Drawing for the job (mm, zero at the part's lowest x, y, z). A direction names the side the tool comes from. Coordinates: 2 decimals unless noted, no trailing zeros. Write each loop counter-clockwise with the first axis right and the second up, starting at its lowest first coordinate (ties: lowest second). Pieces come first, ordered by that corner, then holes. Notation, with made-up numbers: M 56,-28 L 72,-28 A9 ccw 72,-22 Z; hole C 71,1 d4. An arc over 180 degrees is marked long. Put each result on its own line as item: value. Start each with the question number.
Q1. Cut at C-C (y = 3.5). Write the cut outline in (x, z), then the cut area to 3 significant figures.
Q2. Drill centre lines: line 1 along X through (y, z) = (2, 1.75); line 2 along Y through (x, z) = (11.75, 6.5); line 3 along X through (y, z) = (5.75, 5). Where is each one in solid material? Low to high.
Q3. Drop flat-ended pins along their axis: pin 1 (0.6 mm diameter, centred on x = 1, y = 0.5, fed in from -Z); pin 2 (0.6 mm diameter, centred on x = 13.5, z = 9, fed in from +Y); pin 3 (0.8 mm diameter, centred on x = 10, y = 6, fed in from +Z); pin 4 (1.5 mm diameter, centred on y = 1, z = 8.5, fed in from -X). Give the stop position or say it passes through.
Q4. Cut at D-D (z = 8.75). Write the cut outline in (x, y).
Q5. Cut at A-A (x = 13). Write the cut outline in (y, z), then the cut area to 3 significant figures.
Q6. Cut at B-B (z = 2.25). Write the cut outline in (x, y), then the cut area to 3 significant figures.
Q7. Which spindle directions (+Z, -Z, +X, -X, +Y, -Y) get a long thin tool onto all of the face, cutting with end or side? Do the marked faces 1 and 2. Say none if no direction does.
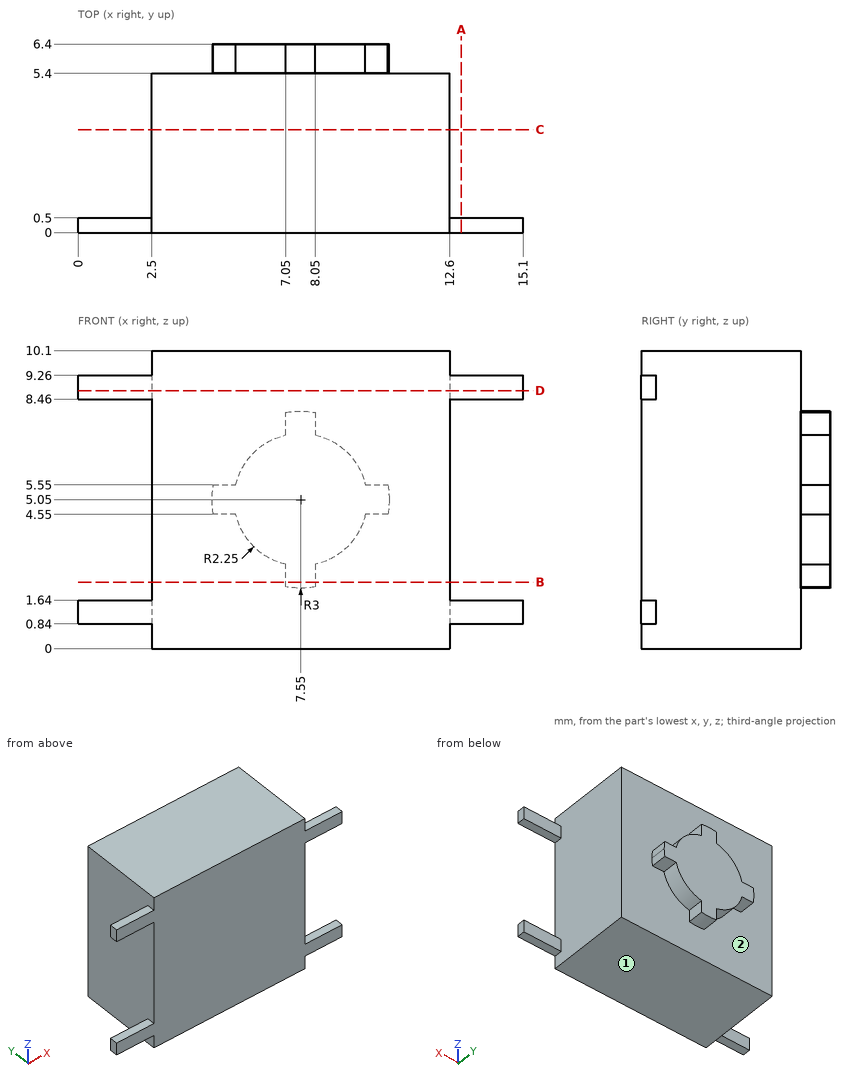
Computed values:
1. outline: M 2.5,0 L 12.6,0 L 12.6,10.1 L 2.5,10.1 Z
1. area: 102 mm2
2. line 1: 2.5 to 12.6
2. line 2: 0 to 5.4
2. line 3: 4.55 to 10.55
3. pin 1: z = 0.84
3. pin 2: y = 0.5
3. pin 3: z = 5.98
3. pin 4: x = 0
4. outline: M 0,0 L 15.1,0 L 15.1,0.5 L 12.6,0.5 L 12.6,5.4 L 2.5,5.4 L 2.5,0.5 L 0,0.5 Z
5. outline: M 0,0.84 L 0.5,0.84 L 0.5,1.64 L 0,1.64 Z; M 0,8.46 L 0.5,8.46 L 0.5,9.26 L 0,9.26 Z
5. area: 0.800 mm2
6. outline: M 2.5,0 L 12.6,0 L 12.6,5.4 L 8.05,5.4 L 8.05,6.4 L 7.05,6.4 L 7.05,5.4 L 2.5,5.4 Z
6. area: 55.5 mm2
7. face 1: -Z, +X, -X, +Y, -Y
7. face 2: +Y
